The listing builds one solid part. Answer for the finished solid, in the listing's coordinates (mm). A direction names the side the tool comes from. Give positions to 0.01 mm unless a question says otherwise; leave off trailing zeros. Order: outer loops, then holes, each group sorted by start corner. A loop starts at its lowest first (then second) coordinate and runs counter-clockwise, first axis right, second up. Notation, with made-up numbers: (8.25, 78) - (26.25, 78) arc R20 cw to (26.25, 117) - close; hole circle Ø5 at (88, 15.25). An arc over 180 degrees is marked (long way). Answer in a Markdown table with one row per item. Add a question column.
```python
from build123d import *

# Parameters (mm, degrees)
F1_DEPTH = 12
F0_R     = 2
F2_DEPTH = 5.2
F3_SIZE  = 1
F4_R     = 4.15
F5_DEPTH = 8
F6_R     = 3
F7_DEPTH = 3


with BuildPart() as f1:
    # F0 (on Top) → F1 (new body)
    with BuildSketch(Plane.XY):
        Polygon((14.7, 8.5), (-14.7, 8.5), (-19, 4.2), (-19, -4.2), (-14.7, -8.5), (14.7, -8.5), (19, -4.2), (19, 4.2), align=None)
    extrude(amount=F1_DEPTH)

    # F0 (on Top) → F2 (join)
    with BuildSketch(Plane.XY):
        Polygon((22.5, 11.5), (-22.5, 11.5), (-28.5, 5.5), (-28.5, -5.5), (-22.5, -11.5), (22.5, -11.5), (28.5, -5.5), (28.5, 5.5), align=None)
        with Locations((-24.75, 0)):
            Circle(F0_R, mode=Mode.SUBTRACT)
        Polygon((-19, 4.2), (-14.7, 8.5), (14.7, 8.5), (19, 4.2), (19, -4.2), (14.7, -8.5), (-14.7, -8.5), (-19, -4.2), align=None, mode=Mode.SUBTRACT)
        with Locations((24.75, 0)):
            Circle(F0_R, mode=Mode.SUBTRACT)
    extrude(amount=F2_DEPTH)

    # F3
    f3_edges = [f1.edges().sort_by_distance(p)[0] for p in [
        (0, -11.5, 0),
        (-25.5, -8.5, 0),
        (-28.5, 0, 0),
        (-25.5, 8.5, 0),
        (0, 11.5, 0),
        (25.5, 8.5, 0),
        (28.5, 0, 0),
        (25.5, -8.5, 0),
    ]]
    chamfer(f3_edges, length=F3_SIZE)

    # F4 (on face) → F5 (cut)
    with BuildSketch(Plane.XY.offset(12)):
        Circle(F4_R)
    extrude(amount=-F5_DEPTH, mode=Mode.SUBTRACT)

    # F6 (on Top) → F7 (cut)
    with BuildSketch(Plane.XY):
        with Locations((-23.793586, 0)):
            Circle(F6_R)
        with Locations((23.756452, 0)):
            Circle(F6_R)
    extrude(amount=F7_DEPTH, mode=Mode.SUBTRACT)


solid = f1.part
```
(1) Find section D-D, the plane x = 0. Write down the section's boundary in (y, z), plus the area to 3 significant figures.
(2) For faces 4 (the face through (0, 8.5, 9)), 5 (the face through (-25, 9, 3)), 6 (the face through (20.76, 0.13, 1.48)), 7 (the face through (-16.8, 6.4, 8.6)), 8 (the face through (19, 0, 9)), determine the directions among +Z, -Z, +X, -X, +Y, -Y from which every point of the face is accessible in a straight line to the end or side of a thin tool.
(3) The mould has two halves that part along X. Classify faces 1 (the face through (22, 0, 3)), 2 (the face through (25, -9, 3)), 3 (the face through (0, -10, 5.2)): +X half, -X half, draft (parallel to the pull), parting line (faces both ways), or undercut.
(4) Find section A-A, the plane z = 10. Write down the section's boundary in (x, y), plus the area to 3 significant figures.
(5) Find section C-C, the plane y = 0. Give the number of separate pieces and of enclosed holes in the cut face, plus the area to 3 significant figures.
(6) Each of these flat-tipped pins is pushed along its axis until it touches: P1, Ø3, axis at x = 23.5, y = -1, coming from the -Z side; P2, Ø4, axis at y = -4, z = 9.5, coming from the +X side; P3, Ø7, axis at x = 23.76, y = 0, coming from the +Z side. Where does it stop, or does it pass through?
(7) Find section B-B, the plane x = 24.75. Write down the section's boundary in (y, z), plus the area to 3 significant figures.
(8) Straight lines are drawn through the part: line 1 (X direction, y = 0, z = 3.9); line 2 (Y direction, x = 0, z = 7); line 3 (X direction, y = 0.25, z = 6). For each, find the intervals that lie inside material, in ascending order.
Answer key:
| question | item | result |
|---|---|---|
| 1 | outline | (-11.5, 1) - (-10.5, 0) - (10.5, 0) - (11.5, 1) - (11.5, 5.2) - (8.5, 5.2) - (8.5, 12) - (4.15, 12) - (4.15, 4) - (-4.15, 4) - (-4.15, 12) - (-8.5, 12) - (-8.5, 5.2) - (-11.5, 5.2) - close |
| 1 | area | 168 mm² |
| 2 | face 4 | +Z, +X, -X, +Y |
| 2 | face 5 | +Z, -Z, -X, +Y |
| 2 | face 6 | -Z |
| 2 | face 7 | +Z, -X, +Y |
| 2 | face 8 | +Z, +X, +Y, -Y |
| 3 | face 1 | undercut |
| 3 | face 2 | +X half |
| 3 | face 3 | draft |
| 4 | outline | (-19, -4.2) - (-14.7, -8.5) - (14.7, -8.5) - (19, -4.2) - (19, 4.2) - (14.7, 8.5) - (-14.7, 8.5) - (-19, 4.2) - close; hole circle Ø8.3 at (0, 0) |
| 4 | area | 555 mm² |
| 5 | separate pieces | 3 |
| 5 | enclosed holes | 0 |
| 5 | area | 434 mm² |
| 6 | P1 | z = 3 |
| 6 | P2 | x = 19 |
| 6 | P3 | z = 5.2 |
| 7 | outline | (-9.25, 1) - (-7.84, 0) - (-2.83, 0) - (-2.83, 3) - (-2, 3) - (-2, 5.2) - (-9.25, 5.2) - close; (2, 3) - (2.83, 3) - (2.83, 0) - (7.84, 0) - (9.25, 1) - (9.25, 5.2) - (2, 5.2) - close |
| 7 | area | 69.0 mm² |
| 8 | line 1 | -28.5 to -26.75, -22.75 to 22.75, 26.75 to 28.5 |
| 8 | line 2 | -8.5 to -4.15, 4.15 to 8.5 |
| 8 | line 3 | -19 to -4.14, 4.14 to 19 |
